```python
from build123d import *

# Parameters (mm, degrees)
SKETCH_W     = 40
SKETCH_H     = 40
PAD_DEPTH    = 3.5
SKETCH001_R  = 2.5
POCKET_DEPTH = 5
SKETCH002_R  = 3.5
PAD001_DEPTH = 125
PAD002_DEPTH = 10


with BuildPart() as part:
    # Sketch → Pad (new body)
    with BuildSketch(Plane.XY):
        Rectangle(SKETCH_W, SKETCH_H)
    extrude(amount=PAD_DEPTH)

    # Sketch001 (on Face6 of Pad) → Pocket (cut)
    with BuildSketch(Plane.XY.offset(3.5)):
        with Locations((-10, 10)):
            Circle(SKETCH001_R)
        with Locations((10, -10)):
            Circle(SKETCH001_R)
    extrude(amount=-POCKET_DEPTH, mode=Mode.SUBTRACT)

    # Sketch002 (on Face1 of Pocket) → Pad001 (join)
    with BuildSketch(Plane(origin=(0, 20, 0), x_dir=(-1, 0, 0), z_dir=(0, 1, 0))):
        with Locations((0, 3.5)):
            Circle(SKETCH002_R)
    extrude(amount=PAD001_DEPTH)

    # Sketch003 (on Face11 of Pad001) → Pad002 (join)
    with BuildSketch(Plane.XZ.offset(-20)):
        with BuildLine():
            ThreePointArc((3.5, 3.5), (0, 7), (-3.5, 3.5))
            Line((-3.5, 3.5), (3.5, 3.5))
        make_face()
    extrude(amount=PAD002_DEPTH)


solid = part.part
```
Can you work these out from the model? Positions are in its coordinate system, mm. A direction names the side the tool comes from. Round coordinates to 2 decimals unless told otherwise and drop trailing zeros. Order: outer loops, then holes, each group sorted by start corner. A loop starts at its lowest first (then second) coordinate and runs counter-clockwise, first axis right, second up.
(1) On a 3-axis mill with a long thin cutter (end or side, diameter ignored), from which of +Z, -Z, +X, -X, +Y, -Y can I reach the whole of each face in a straight line? I mean faces 5 (the face through (0, 10, 5)), 6 (the face through (0, 145, 4)). Say none if no direction works.
Results are:
face 5: +Z, +X, -X, -Y
face 6: +Z, -Z, +X, -X, +Y
(2) I'm going to push flat-ended pins straight in: pin 1 (1.8 mm diameter, centred on x = -7, z = 1.5, fed in from +Y); pin 2 (4.5 mm diameter, centred on x = 10, y = -10, fed in from -Z); pin 3 (1.5 mm diameter, centred on y = 93.5, z = 6, fed in from +X); pin 4 (4 mm diameter, centred on x = -1.5, z = 6, fed in from -Y). Where does each tip first touch, or does it pass through?
Results are:
pin 1: stops at y = 20
pin 2: passes through
pin 3: stops at x = 3.03
pin 4: stops at y = 10
(3) If we section it at A-A (x = -10): Please give me the cut outline in (y, z).
Results are:
outline: (-20, 0) - (7.5, 0) - (7.5, 3.5) - (-20, 3.5) - close; (12.5, 0) - (20, 0) - (20, 3.5) - (12.5, 3.5) - close
(4) If I drill on L1, parallel to Y at x = 10, z = 2.6; L2, parallel to Y at x = 5.5, z = 3.25; L3, parallel to Z at x = -4.5, y = -4, over which ranges is the centre line in solid material (lowest first)?
Results are:
L1: y = -20 to -12.5, -7.5 to 20
L2: y = -20 to 20
L3: z = 0 to 3.5
(5) We'd pull the mould along Y, two halves only. Please class faces 1 (the face through (12, 20, 2)), 2 (the face through (9.46, -12.44, 1.77)), 3 (the face through (20, 0, 2)), 4 (the face through (0, -20, 2)): +Y half, -Y half, draft (parallel to the pull), parting line (faces both ways), or undercut.
Results are:
face 1: +Y half
face 2: undercut
face 3: draft
face 4: -Y half
(6) If we section it at B-B (x = -2): Please give me the cut outline in (y, z).
Results are:
outline: (-20, 0) - (20, 0) - (20, 0.63) - (145, 0.63) - (145, 6.37) - (10, 6.37) - (10, 3.5) - (-20, 3.5) - close
(7) If we section it at C-C (y = 45.5): Please give me the cut outline in (x, z), plus the area to 3 significant figures.
Results are:
outline: circle Ø7 at (0, 3.5)
area: 38.5 mm2
